Design review of the part shown in the three views and the two pictorial views. Dimensions are in mm from the part's minimum x, y and z. A direction names the side the tool comes from. Coordinates: 2 decimals unless noted, no trailing zeros. Write each loop counter-clockwise with the first axis right and the second up, starting at its lowest first coordinate (ties: lowest second). Pieces come first, ordered by that corner, then holes. Notation, with made-up numbers: M -33.5,-23 L 21.5,-23 A14 ccw 21.5,-3 Z; hole C 42.5,19 d5. An arc over 180 degrees is marked long. Answer as a JSON object with one key per item and string values.
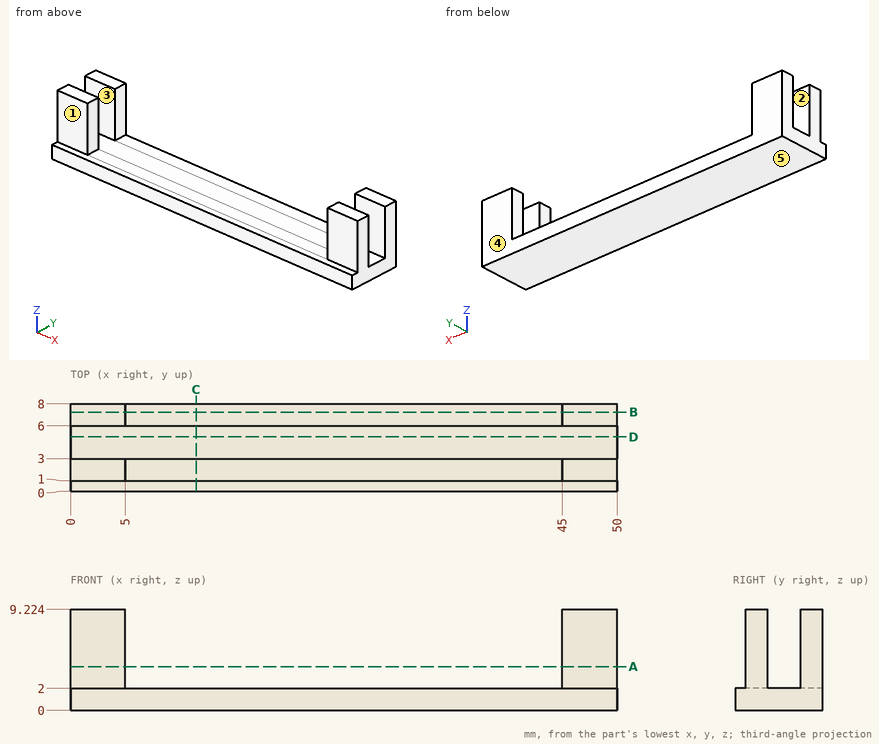
(1) Add section C-C on x = 11.5. Give the boundary of the cut face in (y, z), and give its area (3 significant figures).
Results list:
{"outline": "M 0,0 L 8,0 L 8,2 L 0,2 Z", "area": "16.0 mm²"}
(2) Add section A-A on z = 4. Give the boundary of the cut face in (x, y), and give its area (3 significant figures).
Results list:
{"outline": "M 0,1 L 5,1 L 5,3 L 0,3 Z; M 0,6 L 5,6 L 5,8 L 0,8 Z; M 45,1 L 50,1 L 50,3 L 45,3 Z; M 45,6 L 50,6 L 50,8 L 45,8 Z", "area": "40.0 mm²"}
(3) Wall thickness on line 1 along X through (y, z) = (7.5, 5); line 2 along Z through (x, y) = (10, 1.25); line 3 along Y through (x, z) = (46.5, 8): over which ranges is each line inside the solid? List them lowest first. Write a range as from..to.
Results list:
{"line 1": "0..5, 45..50", "line 2": "0..2", "line 3": "1..3, 6..8"}
(4) Draft analysis for pull direction Y (two halves, no side actions). For the marked faces 3, 4 and 5, state which applies: released by +Y, released by -Y, zero draft, split by the parting line, or undercut.
Results list:
{"face 3": "undercut", "face 4": "released by +Y", "face 5": "zero draft"}
(5) Add section B-B on y = 7.25. Give the boundary of the cut face in (x, z), and give its area (3 significant figures).
Results list:
{"outline": "M 0,0 L 50,0 L 50,9.22 L 45,9.22 L 45,2 L 5,2 L 5,9.22 L 0,9.22 Z", "area": "172 mm²"}
(6) Add section D-D on y = 5. Give the boundary of the cut face in (x, z), and give its area (3 significant figures).
Results list:
{"outline": "M 0,0 L 50,0 L 50,2 L 0,2 Z", "area": "100 mm²"}
(7) For pin 1 Ø1.5 at (x, y) = (20.5, 4) entering from +Z, flat-tipped, find the tip position at first contact; note if it passes through.
Results list:
{"pin 1": "z = 2"}
(8) For the marked faces 1 and 2, list the 3-axis set-ups (+Z, -Z, +X, -X, +Y, -Y) from which the entire face can be reached by the end or side of a thin tool; tool diameter is ignored.
Results list:
{"face 1": "+Z, +X, -X, -Y", "face 2": "+Z, +X, -X"}
